Here's the drawing with two shaded views (mm, measured from the low corner). I have some questions. A direction names the side the tool comes from. Round coordinates to 2 decimals unless told otherwise and drop trailing zeros. Write each loop counter-clockwise with the first axis right and the second up, starting at its lowest first coordinate (ties: lowest second). Pieces come first, ordered by that corner, then holes. Notation, with made-up numbers: M 0.25,23.25 L 33.25,23.25 A18 ccw 33.25,31.25 Z; hole C 78,25.5 d5. An arc over 180 degrees is marked long. Answer as a JSON object with one key per item and string values. Group by question number.
1) Suppose I cut it at A-A, the plane y = 13.75. Write out the boundary of the cut face in (x, z), and give its area (3 significant figures).
2) Suppose I cut it at B-B, the plane z = 5.5. Write out the boundary of the cut face in (x, y).
3) I'm going to push flat-ended pins straight in: pin 1 Ø1.2 at (x, y) = (14.5, 3.5) entering from +Z; pin 2 Ø1.2 at (x, y) = (3.5, 14.5) entering from -Z; pin 3 Ø1.2 at (x, z) = (25.5, 5) entering from -Y. Where does each tip first touch, or does it pass through?
4) On a 3-axis mill with a long thin cutter (end or side, diameter ignored), from which of +Z, -Z, +X, -X, +Y, -Y can I reach the whole of each face in a straight line? I mean the marked faces 1, 2, 3, 4 and 5. Say none if no direction works.
5) Suppose I cut it at C-C, the plane x = 3. Write out the boundary of the cut face in (y, z).
6) Please list where these lines run through material, in increasing order: L1, parallel to Z at x = 15, y = 1.75; L2, parallel to Y at x = 13.75, z = 17. Write a range as [from, to].
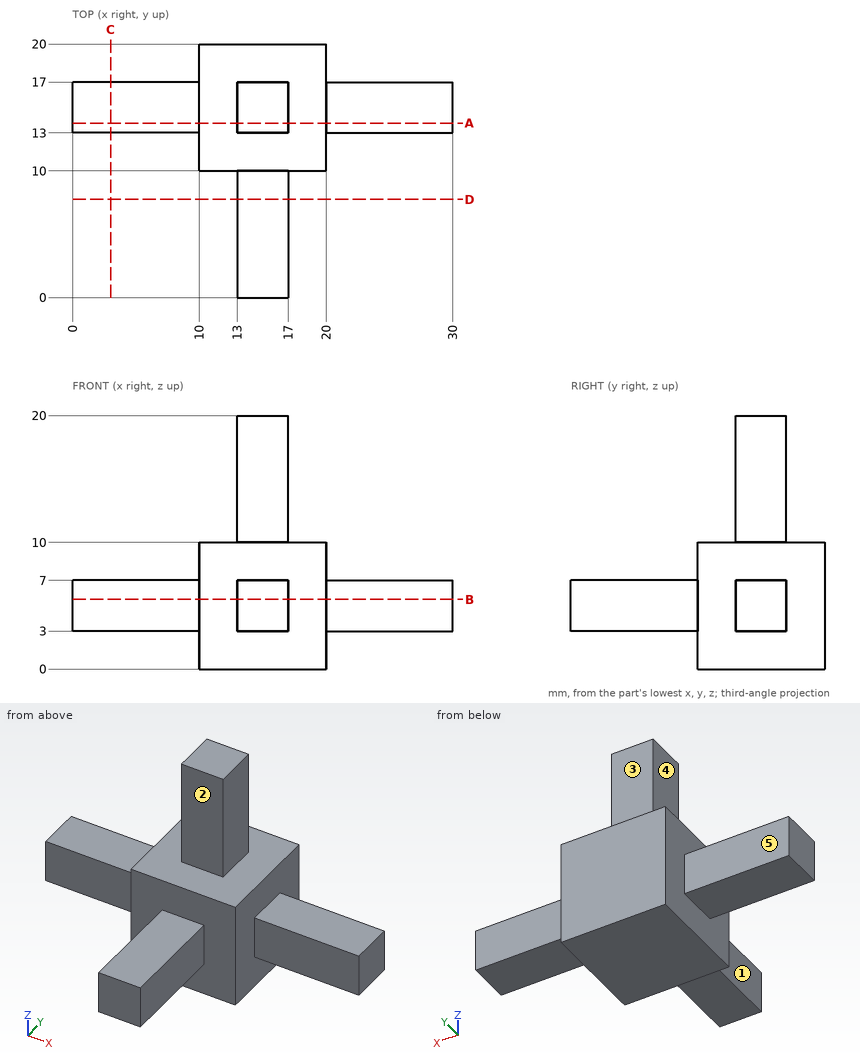
Results:
{
 "1": {"outline": "M 0,3 L 10,3 L 10,0 L 20,0 L 20,3 L 30,3 L 30,7 L 20,7 L 20,10 L 17,10 L 17,20 L 13,20 L 13,10 L 10,10 L 10,7 L 0,7 Z", "area": "220 mm^2"},
 "2": {"outline": "M 0,13 L 10,13 L 10,10 L 13,10 L 13,0 L 17,0 L 17,10 L 20,10 L 20,13 L 30,13 L 30,17 L 20,17 L 20,20 L 10,20 L 10,17 L 0,17 Z"},
 "3": {"pin 1": "z = 7", "pin 2": "z = 3", "pin 3": "y = 13"},
 "4": {"face 1": "+Z, -Z, -X, -Y", "face 2": "+Z, +X, -X, -Y", "face 3": "+Z, +X, -X, +Y", "face 4": "+Z, -X, +Y, -Y", "face 5": "+Z, -Z, -X, +Y"},
 "5": {"outline": "M 13,3 L 17,3 L 17,7 L 13,7 Z"},
 "6": {"L1": "[3, 7]", "L2": "[13, 17]"}
}
